Answer from the drawing. Dimensions are ordinates in mm from the lowest x, y and z of the part. Round coordinates to 2 decimals unless told otherwise and drop trailing zeros. Loops run counter-clockwise (first coordinate to the right, second up) from the corner with the lowest first, then second, coordinate; pieces in that order, holes last. Notation, with made-up numbers: M 13.25,45 L 70.25,45 A19 cw 70.25,52 Z; hole C 80,77 d8. An arc over 180 degrees is marked long. One line per item, written item: value.
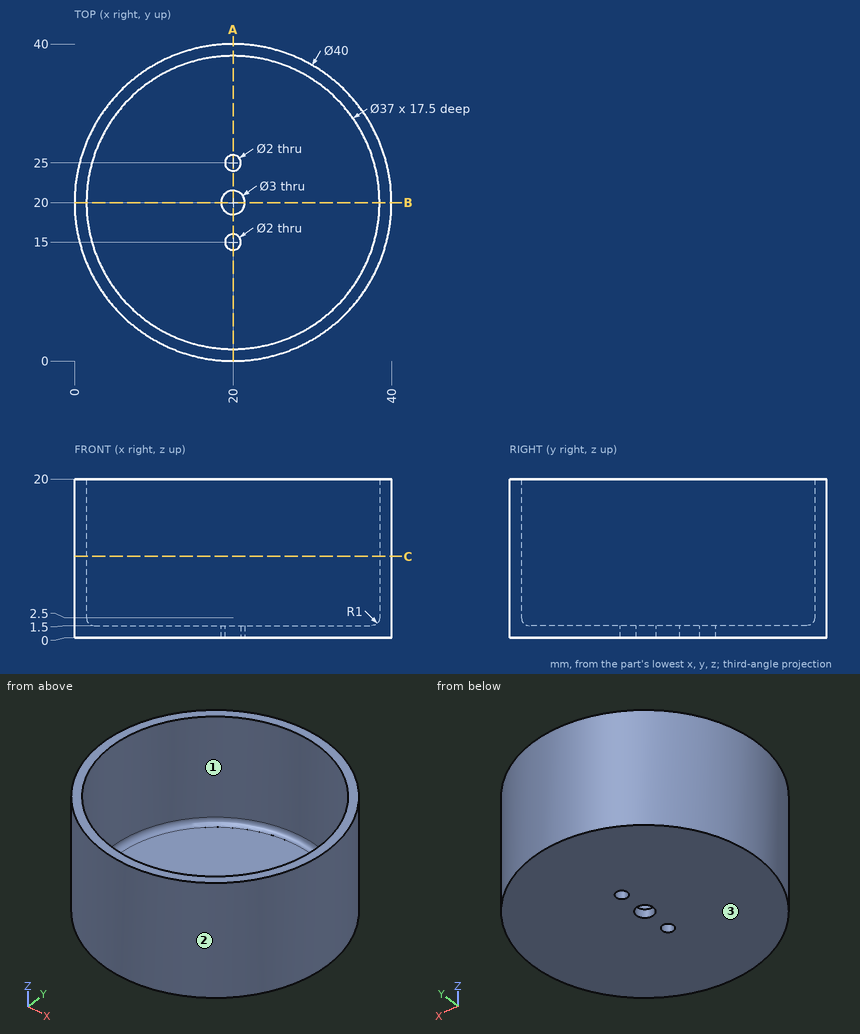
1) Find section B-B (y = 20). Give the vertices of the cut face in (x, z).
Check values:
outline: M 0,0 L 18.5,0 L 18.5,1.5 L 2.5,1.5 A1 cw 1.5,2.5 L 1.5,20 L 0,20 Z; M 21.5,0 L 40,0 L 40,20 L 38.5,20 L 38.5,2.5 A1 cw 37.5,1.5 L 21.5,1.5 Z
2) Find the intervals of material crossed by probe 1 along Y at (x, z) = (20, 0.3); probe 2 along X at (y, z) = (20, 15.5), in increasing order. Write a range as from..to.
Check values:
probe 1: 0..14, 16..18.5, 21.5..24, 26..40
probe 2: 0..1.5, 38.5..40
3) Each of these flat-tipped pins is pushed along its axis until it touches: pin 1 (10.5 mm diameter, centred on x = 28, y = 17, fed in from +Z); pin 2 (6 mm diameter, centred on y = 32.5, z = 10.5, fed in from -X); pin 3 (4 mm diameter, centred on y = 34.5, z = 17, fed in from -X). Where does it stop, or does it pass through?
Check values:
pin 1: z = 1.5
pin 2: x = 2.4
pin 3: x = 4.39
4) The mould has two halves that part along Y. Classify the marked faces 1, 2 and 3: +Y half, -Y half, draft (parallel to the pull), parting line (faces both ways), or undercut.
Check values:
face 1: undercut
face 2: parting line
face 3: draft
5) Find section A-A (x = 20). Give the vertices of the cut face in (y, z).
Check values:
outline: M 0,0 L 14,0 L 14,1.5 L 2.5,1.5 A1 cw 1.5,2.5 L 1.5,20 L 0,20 Z; M 16,0 L 18.5,0 L 18.5,1.5 L 16,1.5 Z; M 21.5,0 L 24,0 L 24,1.5 L 21.5,1.5 Z; M 26,0 L 40,0 L 40,20 L 38.5,20 L 38.5,2.5 A1 cw 37.5,1.5 L 26,1.5 Z
6) Find section C-C (z = 10.25). Give the vertices of the cut face in (x, y), then the cut area to 3 significant figures.
Check values:
outline: C 20,20 d40; hole C 20,20 d37
area: 181 mm2
